The listing builds one solid part. Answer for the finished solid, in the listing's coordinates (mm). A direction names the side the tool comes from. Round coordinates to 2 decimals unless told otherwise and drop trailing zeros. Order: outer loops, then holes, each group sorted by start corner. A loop starts at its lowest first (then second) coordinate and runs counter-clockwise, first axis right, second up. Notation, with made-up numbers: M 62.5,13 L 96.5,13 A12 cw 96.5,36 Z; hole C 35,62 d11. An arc over 180 degrees is marked long. Put each result on its own line as item: value. Start each with the question number.
1. Consider line 1 (X direction, y = 0, z = -7); line 2 (Z direction, x = 3, y = -1.75). Determine where each line is inside the solid, lowest interval first.
2. The part is cut by section D-D (y = 4.25). Give the vertices of the cut face in (x, z).
3. Which of the six approach directions +Z, -Z, +X, -X, +Y, -Y give full straight-line access (tool end or side, diameter ignored) to faces 4 (the face through (-1.6, 1.2, -9.2)), 5 (the face through (-0.75, -5.7, -11.83))?
4. The mould has two halves that part along X. Classify faces 1 (the face through (3.807, -0.546, -17.549)), 2 (the face through (5.22, 2.96, 2.96)), 3 (the face through (0, -6, 3)): +X half, -X half, draft (parallel to the pull), parting line (faces both ways), or undercut.
5. The part is cut by section B-B (y = 1.25). Give the vertices of the cut face in (x, z).
6. Each of these flat-tipped pins is pushed along its axis until it touches: pin 1 Ø1 at (y, z) = (1.5, -6.5) entering from -X; pin 2 Ø1.5 at (y, z) = (-4, -4) entering from -X; pin 3 Ø3 at (y, z) = (-4, -3.5) entering from -X. Where does it stop, or does it pass through?
7. The part is cut by section C-C (z = -12.5). Give the vertices of the cut face in (x, y).
8. The part is cut by section A-A (x = 0). Give the vertices of the cut face in (y, z), then the cut area to 3 significant figures.
from build123d import *

# Parameters (mm, degrees)
BOSS_EXTRUDE1_DEPTH = 6
SKETCH2_R           = 5.75
BOSS_EXTRUDE2_DEPTH = 24
SKETCH4_R           = 2
CUT_EXTRUDE2_DEPTH  = 31
SKETCH5_R           = 1.5
CUT_EXTRUDE3_DEPTH  = 6


with BuildPart() as part:
    # Sketch1 → Boss-Extrude1 (new body)
    with BuildSketch(Plane(origin=(0, 0, 0), x_dir=(0, 1, 0), z_dir=(0, 0, 1))):
        Polygon((0, 6.92820323), (-6, 3.464101615), (-6, -3.464101615), (0, -6.92820323), (6, -3.464101615), (6, 3.464101615), align=None)
    extrude(amount=BOSS_EXTRUDE1_DEPTH)

    # Sketch2 → Boss-Extrude2 (add)
    with BuildSketch(Plane(origin=(0, 0, 0), x_dir=(1, 0, 0), z_dir=(0, 0, -1))):
        Circle(SKETCH2_R)
    extrude(amount=BOSS_EXTRUDE2_DEPTH)

    # Sketch4 → Cut-Extrude2 (cut, through all)
    with BuildSketch(Plane(origin=(0, 0, -24), x_dir=(1, 0, 0), z_dir=(0, 0, -1))):
        Circle(SKETCH4_R)
    extrude(amount=-CUT_EXTRUDE2_DEPTH, mode=Mode.SUBTRACT)

    # Sketch5 → Cut-Extrude3 (cut)
    with BuildSketch(Plane(origin=(5.196152423, -3, 0), x_dir=(0.5, 0.866025404, 0), z_dir=(0.866025404, -0.5, 0))):
        with Locations((0, -18)):
            Circle(SKETCH5_R)
    extrude(amount=-CUT_EXTRUDE3_DEPTH, mode=Mode.SUBTRACT)


solid = part.part
Resolved:
1. line 1: -5.75 to -2, 2 to 5.75
1. line 2: -24 to -19.5, -16.5 to 6
2. outline: M -4.47,0 L -3.87,0 L -3.87,-24 L 3.87,-24 L 3.87,0 L 4.47,0 L 4.47,6 L -4.47,6 Z
3. face 4: +Z, -Z
3. face 5: -Z
4. face 1: undercut
4. face 2: +X half
4. face 3: draft
5. outline: M -6.21,0 L -5.61,0 L -5.61,-24 L -1.56,-24 L -1.56,6 L -6.21,6 Z; M 1.56,-24 L 5.61,-24 L 5.61,0 L 6.21,0 L 6.21,6 L 1.56,6 Z
6. pin 1: x = -5.66
6. pin 2: x = -4.74
6. pin 3: x = -5.18
7. outline: C 0,0 d11.5; hole C 0,0 d4
8. outline: M -6,0 L -5.75,0 L -5.75,-24 L -2,-24 L -2,6 L -6,6 Z; M 2,-24 L 5.75,-24 L 5.75,0 L 6,0 L 6,6 L 2,6 Z
8. area: 228 mm2
